```python
from build123d import *

# Parameters (mm, degrees)
SKETCH1_R           = 14.3129
BOSS_EXTRUDE1_DEPTH = 6.35
FILLET1_R           = 14.2875
SKETCH2_W           = 38.1
SKETCH2_H           = 44.45
BOSS_EXTRUDE2_DEPTH = 6.35
SKETCH3_R           = 14.3129
CUT_EXTRUDE1_DEPTH  = 110.433918417
SKETCH5_R           = 2.38125
CUT_EXTRUDE3_DEPTH  = 110.433918417
FILLET2_R           = 12.7


with BuildPart() as part:
    # Sketch1 → Boss-Extrude1 (new body)
    with BuildSketch(Plane.XY):
        Polygon((-6.35, -6.35), (63.5, -6.35), (63.5, 44.45), (-63.5, 44.45), (-63.5, -44.45), (-31.75, -44.45), align=None)
        with Locations((-44.45, -25.4)):
            Circle(SKETCH1_R, mode=Mode.SUBTRACT)
        with Locations((35.871852568, 12.7)):
            Circle(SKETCH1_R, mode=Mode.SUBTRACT)
    extrude(amount=BOSS_EXTRUDE1_DEPTH)

    # Fillet1
    fillet1_edges = [part.edges().sort_by_distance(p)[0] for p in [
        (-31.75, -44.45, 3.175),
        (-63.5, -44.45, 3.175),
        (63.5, -6.35, 3.175),
        (-6.35, -6.35, 3.175),
    ]]
    fillet(fillet1_edges, radius=FILLET1_R)

    # Sketch2 → Boss-Extrude2 (add)
    with BuildSketch(Plane.XY.offset(6.35)):
        with Locations((8.89, 66.675)):
            Rectangle(SKETCH2_W, SKETCH2_H)
    extrude(amount=-BOSS_EXTRUDE2_DEPTH)

    # Sketch3 → Cut-Extrude1 (cut, through all)
    with BuildSketch(Plane.XY.offset(6.35)):
        with Locations((9.062967637, 68.577618639)):
            Circle(SKETCH3_R)
    extrude(amount=-CUT_EXTRUDE1_DEPTH, mode=Mode.SUBTRACT)

    # Sketch5 → Cut-Extrude3 (cut, through all)
    with BuildSketch(Plane.XY.offset(6.35)):
        with Locations((-15.875, 15.875)):
            Circle(SKETCH5_R)
        with Locations((9.525, 15.875)):
            Circle(SKETCH5_R)
    extrude(amount=-CUT_EXTRUDE3_DEPTH, mode=Mode.SUBTRACT)

    # Fillet2
    fillet2_edges = [part.edges().sort_by_distance(p)[0] for p in [
        (-10.16, 44.45, 3.175),
        (-10.16, 88.9, 3.175),
        (27.94, 88.9, 3.175),
        (27.94, 44.45, 3.175),
    ]]
    fillet(fillet2_edges, radius=FILLET2_R)


solid = part.part
```
CAD build for the part. Positions are in the model's coordinates, mm. A direction names the side the tool comes from. Round coordinates to 2 decimals unless told otherwise and drop trailing zeros. Write each loop counter-clockwise with the first axis right and the second up, starting at its lowest first coordinate (ties: lowest second). Pieces come first, ordered by that corner, then holes.
Item 1: Mould opens along Y. For faces 6 (the cylindrical face through (59.2, -2.28, 3.22)), 7 (the flat face through (9, 88.9, 3)), 8 (the cylindrical face through (7.77, 17.484, 3.219)) say: released by +Y, released by -Y, zero draft, split by the parting line, or undercut.
Filled in:
face 6: released by -Y
face 7: released by +Y
face 8: undercut
Item 2: Drop flat-ended pins along their axis: pin 1 Ø7.5 at (x, y) = (-15.875, 15.875) entering from +Z; pin 2 Ø3 at (x, y) = (9.525, 15.875) entering from +Z; pin 3 Ø3 at (y, z) = (71, 3) entering from +X; pin 4 Ø3 at (y, z) = (63, 4) entering from -X. Give the stop position or say it passes through.
Filled in:
pin 1: stops at z = 6.35
pin 2: passes through
pin 3: stops at x = 27.94
pin 4: stops at x = -10.16
Item 3: Band-saw the part on A-A on y = -25.4. Write the cut outline in (x, z).
Filled in:
outline: (-63.5, 0) - (-58.76, 0) - (-58.76, 6.35) - (-63.5, 6.35) - close; (-30.14, 0) - (-19.05, 0) - (-19.05, 6.35) - (-30.14, 6.35) - close
Item 4: Band-saw the part on D-D on y = 51. Write the cut outline in (x, z), then the cut area to 3 significant figures.
Filled in:
outline: (-11.75, 0) - (29.53, 0) - (29.53, 6.35) - (-11.75, 6.35) - close
area: 262 mm2
Item 5: Drill centre lines: L1, parallel to X at y = 68, z = 5.5; L2, parallel to X at y = -34, z = 3.75 (3 decimals); L3, parallel to Y at x = -32.5, z = 0.5. Where is each one in solid material? Low to high.
Filled in:
L1: x = -10.16 to -5.24, 23.36 to 27.94
L2: x = -62.975 to -55.891, -33.009 to -24.783
L3: y = -42.68 to -33.28, -17.52 to 44.45
Item 6: Band-saw the part on C-C on z = 3. Give the number of separate pieces and of enclosed holes in the cut face, then the cut area to 3 significant figures.
Filled in:
separate pieces: 1
enclosed holes: 5
area: 7,780 mm2
Item 7: Tool access for faces 1 (the flat face through (52, 44.45, 3)), 2 (the cylindrical face through (-13.604, 16.59, 3.219)), 3 (the cylindrical face through (-59.2, -40.38, 3.22)), 4 (the flat face through (25, -6.35, 3)), 5 (the flat face through (-43, 44.45, 3)): list every direction of +Z, -Z, +X, -X, +Y, -Y with a clear straight run to the whole face (end or side of a thin tool).
Filled in:
face 1: +Z, -Z, +X, +Y
face 2: +Z, -Z
face 3: +Z, -Z, -X, -Y
face 4: +Z, -Z, +X, -Y
face 5: +Z, -Z, -X, +Y
Item 8: Band-saw the part on B-B on x = -44.45. Write the cut outline in (y, z).
Filled in:
outline: (-44.45, 0) - (-39.71, 0) - (-39.71, 6.35) - (-44.45, 6.35) - close; (-11.09, 0) - (44.45, 0) - (44.45, 6.35) - (-11.09, 6.35) - close
